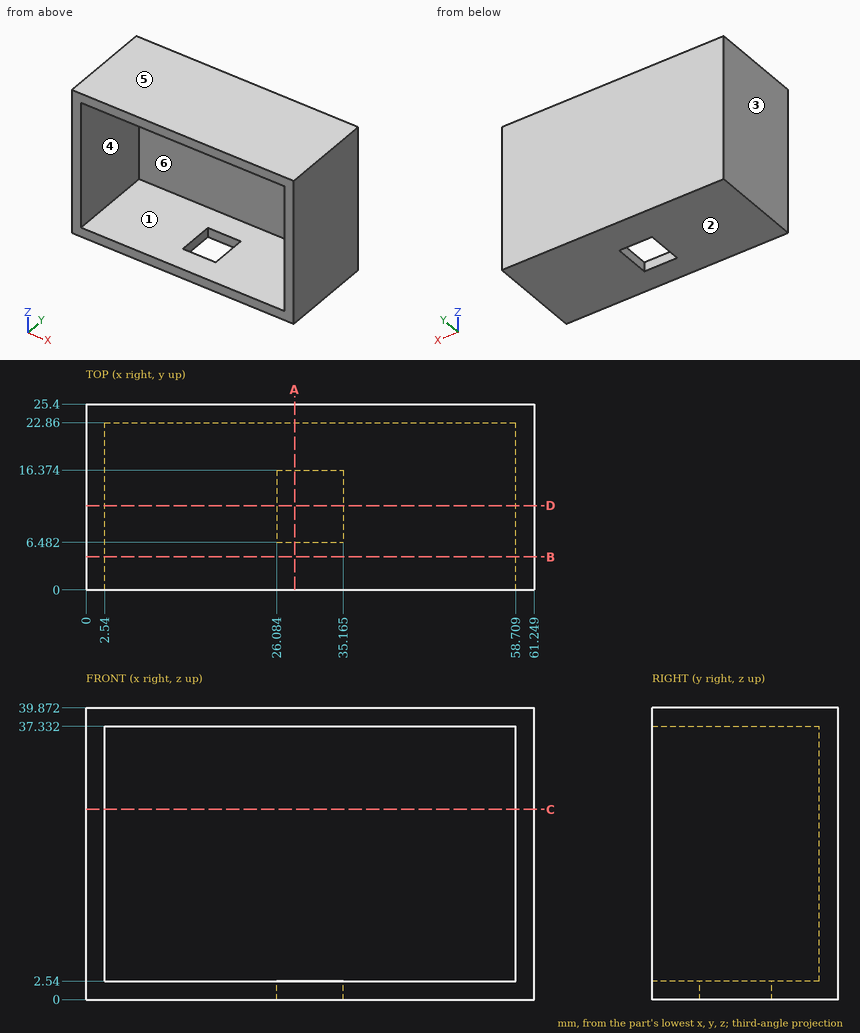
Source: three-view drawing plus pictorial views. Frame: mm from the lowest corner of the part. A direction names the side the tool comes from. Give positions to 0.01 mm unless a question says otherwise; leave off trailing zeros. Order: outer loops, then holes, each group sorted by start corner. A loop starts at its lowest first (then second) coordinate and runs counter-clockwise, first axis right, second up. Notation, with made-up numbers: M 24,-38 L 49,-38 A33 cw 49,-8 Z; hole C -10,46.5 d7. An arc over 180 degrees is marked long. Return JSON: item names as keys, results as strings.
Item 1: Ray query, probe 1 along Z at (x, y) = (47, 21.5); probe 2 along X at (y, z) = (20.5, 16.5); probe 3 along Y at (x, z) = (36, 37). Return the intervals inside material, ascending.
Solutions:
{"probe 1": "0 to 2.54, 37.33 to 39.87", "probe 2": "0 to 2.54, 58.71 to 61.25", "probe 3": "22.86 to 25.4"}
Item 2: Access query for the marked faces 1 and 2. Directions: +Z, -Z, +X, -X, +Y, -Y. A direction counts if a zero-diameter tool reaches every point of the face in a straight line with its end or side. Return the directions, or none.
Solutions:
{"face 1": "-Y", "face 2": "-Z, +X, -X, +Y, -Y"}
Item 3: First-contact query: P1, Ø1.5, axis at x = 18.5, z = 29, coming from the -Y side. Flat tip, straight axial feed; report the tip coordinate or a pass-through.
Solutions:
{"P1": "y = 22.86"}
Item 4: Pull-direction query (Z, two-part tool) for the marked faces 3, 4, 5 and 6; classes: +Z half, -Z half, draft (parallel to the pull), parting line (faces both ways), or undercut.
Solutions:
{"face 3": "draft", "face 4": "undercut", "face 5": "+Z half", "face 6": "undercut"}
Item 5: Cut plane A-A (x = 28.5). Return loops of the section in (y, z).
Solutions:
{"outline": "M 0,0 L 6.48,0 L 6.48,2.54 L 0,2.54 Z; M 0,37.33 L 22.86,37.33 L 22.86,2.54 L 16.37,2.54 L 16.37,0 L 25.4,0 L 25.4,39.87 L 0,39.87 Z"}
Item 6: Cut plane C-C (z = 26). Return loops of the section in (x, y), then the cut area to 3 significant figures.
Solutions:
{"outline": "M 0,0 L 2.54,0 L 2.54,22.86 L 58.71,22.86 L 58.71,0 L 61.25,0 L 61.25,25.4 L 0,25.4 Z", "area": "272 mm^2"}
Item 7: Cut plane D-D (y = 11.5). Return loops of the section in (x, z) (1 decimal), then the cut area to 3 significant figures.
Solutions:
{"outline": "M 0,0 L 26.1,0 L 26.1,2.5 L 2.5,2.5 L 2.5,37.3 L 58.7,37.3 L 58.7,2.5 L 35.2,2.5 L 35.2,0 L 61.2,0 L 61.2,39.9 L 0,39.9 Z", "area": "465 mm^2"}
Item 8: Cut plane B-B (y = 4.5). Return loops of the section in (x, z).
Solutions:
{"outline": "M 0,0 L 61.25,0 L 61.25,39.87 L 0,39.87 Z; hole M 2.54,2.54 L 58.71,2.54 L 58.71,37.33 L 2.54,37.33 Z"}
